Build history of the part. All positions in model axes, mm. A direction names the side the tool comes from. Give positions to 0.01 mm unless a question says otherwise; leave off trailing zeros. Loops run counter-clockwise (first coordinate to the right, second up) from the corner with the lowest first, then second, coordinate; pieces in that order, holes last.
1) Band-saw the part on B-B on z = -0.9. List the corners of the cut face in (x, y), then the cut area to 3 significant figures.
2) Band-saw the part on A-A on y = 11.25. List the corners of the cut face in (x, z), then the cut area to 3 significant figures.
3) Two-plate mould, pull along X, no slides. Class faces 4 (the cylindrical face through (-0.596, 21.479, 2.685)), 5 (the flat face through (2, 23, 1)), 6 (the flat face through (0.348, 22.014, 1.715)): +X half, -X half, draft (parallel to the pull), parting line (faces both ways), or undercut.
4) Flat gauge pins, fed straight in: P1, Ø1.5, axis at x = -1.5, y = 19, coming from the -Z side; P2, Ø2, axis at y = 6.5, z = -1.5, coming from the +X side; P3, Ø1.5, axis at y = 13, z = -1.5, coming from the +X side. Where does each tip first touch, or does it go through?
5) Band-saw the part on C-C on x = 1.7. List the corners of the cut face in (y, z).
6) 3-axis set-ups, long thin cutter, end or side, ignore diameter. For faces 1 (the cylindrical face through (-1.5, 9.86, -0.07)), 2 (the flat face through (0, 0, 0)), 3 (the flat face through (-1.31, 22.01, 1.16)): which of +Z, -Z, +X, -X, +Y, -Y reach the whole face in a straight line?
7) Wall check: line 1 (Z direction, x = 0, y = 5.5); line 2 (Y direction, x = -0.3, z = -0.3); line 3 (Y direction, x = -0.75, z = -1.6). Give the ranges that are in metal, low to high.
8) Band-saw the part on D-D on x = 0. List the corners of the cut face in (y, z), then the cut area to 3 significant figures.
```python
from build123d import *

# Parameters (mm, degrees)
SKETCH1_R           = 1.5
BOSS_EXTRUDE1_DEPTH = 20
SKETCH2_R           = 2.75
BOSS_EXTRUDE2_DEPTH = 3
CUT_EXTRUDE1_DEPTH  = 2


with BuildPart() as part:
    # Sketch1 → Boss-Extrude1 (new body)
    with BuildSketch(Plane(origin=(0, 0, 0), x_dir=(1, 0, 0), z_dir=(0, 1, 0))):
        Circle(SKETCH1_R)
    extrude(amount=BOSS_EXTRUDE1_DEPTH)

    # Sketch2 → Boss-Extrude2 (add)
    with BuildSketch(Plane(origin=(0, 20, 0), x_dir=(1, 0, 0), z_dir=(0, 1, 0))):
        Circle(SKETCH2_R)
    extrude(amount=BOSS_EXTRUDE2_DEPTH)

    # Sketch4 → Cut-Extrude1 (cut)
    with BuildSketch(Plane(origin=(0, 23, 0), x_dir=(1, 0, 0), z_dir=(0, 1, 0))):
        Polygon((1.977155875, 0.417358336), (0.627135016, 1.920946383), (-1.350020859, 1.503588046), (-1.977155875, -0.417358336), (-0.627135016, -1.920946383), (1.350020859, -1.503588046), align=None)
    extrude(amount=-CUT_EXTRUDE1_DEPTH, mode=Mode.SUBTRACT)


solid = part.part
```
Findings below:
1. outline: (-2.6, 20) - (-1.2, 20) - (-1.2, 0) - (1.2, 0) - (1.2, 20) - (2.6, 20) - (2.6, 23) - (1.54, 23) - (1.54, 21) - (-1.55, 21) - (-1.55, 23) - (-2.6, 23) - close
1. area: 57.4 mm2
2. outline: circle Ø3 at (0, 0)
2. area: 7.07 mm2
3. face 4: parting line
3. face 5: draft
3. face 6: undercut
4. P1: stops at z = -1.3
4. P2: stops at x = 1.41
4. P3: stops at x = 1.3
5. outline: (20, -2.16) - (23, -2.16) - (23, -0.73) - (21, -0.73) - (21, 0.43) - (23, 0.43) - (23, 2.16) - (20, 2.16) - close
6. face 1: -Y
6. face 2: +Z, -Z, +X, -X, -Y
6. face 3: +Y
7. line 1: z = -1.5 to 1.5
7. line 2: y = 0 to 21
7. line 3: y = 20 to 21
8. outline: (0, -1.5) - (20, -1.5) - (20, -2.75) - (23, -2.75) - (23, -1.79) - (21, -1.79) - (21, 1.79) - (23, 1.79) - (23, 2.75) - (20, 2.75) - (20, 1.5) - (0, 1.5) - close
8. area: 69.3 mm2
